Source: CAD feature listing. Evaluate the final solid. Frame: model axes, mm. A direction names the side the tool comes from. Round coordinates to 2 decimals unless told otherwise and drop trailing zeros. Loops run counter-clockwise (first coordinate to the right, second up) from the corner with the lowest first, then second, coordinate; pieces in that order, holes last. Notation, with made-up numbers: (62, 58.25) -> (98, 58.25) arc R6 cw to (98, 66.25) -> close; hole circle Ø3 at (40, 79.25). An arc over 180 degrees is marked (long way). Write item = value, one per line.
from build123d import *

# Parameters (mm, degrees)
SKETCH009_W             = 100.6
SKETCH009_H             = 82.6
PAD006_DEPTH            = 1.6
SKETCH010_W             = 100.6
SKETCH010_H             = 82.6
SKETCH010_W_2           = 98.6
SKETCH010_H_2           = 80.6
PAD007_DEPTH            = 20.6
SKETCH011_W             = 11.5
SKETCH011_H             = 9
PAD008_DEPTH            = 16.6
SKETCH012_W             = 11.5
SKETCH012_H             = 2
PAD009_DEPTH            = 24.3
SKETCH014_R             = 1.75
POCKET004_DEPTH         = 1.6
SKETCH020_W             = 11.5
SKETCH020_H             = 20
PAD013_DEPTH            = 23.9
BODY003_PLACEMENT_ANGLE = 180


with BuildPart() as part:
    # Sketch009 → Pad006 (new body)
    with BuildSketch(Plane.XY):
        Rectangle(SKETCH009_W, SKETCH009_H)
    extrude(amount=PAD006_DEPTH)

    # Sketch010 → Pad007 (join)
    with BuildSketch(Plane.XY):
        Rectangle(SKETCH010_W, SKETCH010_H)
        Rectangle(SKETCH010_W_2, SKETCH010_H_2, mode=Mode.SUBTRACT)
    extrude(amount=PAD007_DEPTH)

    # Sketch011 → Pad008 (join)
    with BuildSketch(Plane.XY):
        with Locations((-41.95, -27.2)):
            Rectangle(SKETCH011_W, SKETCH011_H)
    extrude(amount=PAD008_DEPTH)

    # Sketch012 → Pad009 (join)
    with BuildSketch(Plane.XY):
        with Locations((-41.95, -21.7)):
            Rectangle(SKETCH012_W, SKETCH012_H)
    extrude(amount=PAD009_DEPTH)

    # Sketch014 → Pocket004 (cut)
    with BuildSketch(Plane.XY):
        with Locations((-45, 36)):
            Circle(SKETCH014_R)
        with Locations((11, 36)):
            Circle(SKETCH014_R)
        with Locations((45, 36)):
            Circle(SKETCH014_R)
        with Locations((45, -36)):
            Circle(SKETCH014_R)
        with Locations((11, -36)):
            Circle(SKETCH014_R)
        with Locations((-45, -36)):
            Circle(SKETCH014_R)
    extrude(amount=POCKET004_DEPTH, mode=Mode.SUBTRACT)

    # Sketch020 → Pad013 (join)
    with BuildSketch(Plane.XY):
        with Locations((-41.95, 21.7)):
            Rectangle(SKETCH020_W, SKETCH020_H)
    extrude(amount=PAD013_DEPTH)


with BuildPart() as part_1:
    # Body003 placement: moved
    add(part.part.moved(Location((0, 0, 57.9))).rotate(Axis((0, 0, 57.9), (1, 0, 0)), BODY003_PLACEMENT_ANGLE))


solid = part_1.part
1. Section query A-A (z = 39). Return the cut outline in (x, y).
Evaluation:
outline = (-50.3, -41.3) -> (50.3, -41.3) -> (50.3, 41.3) -> (-50.3, 41.3) -> close; (-47.7, -31.7) -> (-36.2, -31.7) -> (-36.2, -11.7) -> (-47.7, -11.7) -> close; (-47.7, 20.7) -> (-36.2, 20.7) -> (-36.2, 22.7) -> (-47.7, 22.7) -> close; hole (-49.3, -40.3) -> (49.3, -40.3) -> (49.3, 40.3) -> (-49.3, 40.3) -> close
2. Line query: probe 1 along X at (y, z) = (-20, 39); probe 2 along X at (y, z) = (-36, 57.25); probe 3 along Y at (x, z) = (45, 57.3). Output: solid intervals per line, ascending. Write a range as from..to.
Evaluation:
probe_1 = -50.3..-49.3, -47.7..-36.2, 49.3..50.3
probe_2 = -50.3..-46.75, -43.25..9.25, 12.75..43.25, 46.75..50.3
probe_3 = -41.3..-37.75, -34.25..34.25, 37.75..41.3
3. Set-up query: faces 1 (the face through (-43.383, -35.33, 57.111)), 2 (the face through (-49.3, 1, 47)). Return all of +Z, -Z, +X, -X, +Y, -Y with unobstructed straight access to the full face (end or side cutting, diameter ignored); none if empty.
Evaluation:
face_1 = +Z, -Z
face_2 = -Z
4. Mould query, pull axis X, two halves, no side actions, for faces 3 (the face through (-1, -1, 56.3)), 4 (the face through (50.3, 1, 48)), 5 (the face through (-1, 41.3, 48)). Classes: released by +X, released by -X, zero draft, split by the parting line, or undercut.
Evaluation:
face_3 = undercut
face_4 = released by +X
face_5 = zero draft
5. Section query C-C (y = -36). Return the cut outline in (x, z).
Evaluation:
outline = (-50.3, 37.3) -> (-49.3, 37.3) -> (-49.3, 56.3) -> (-46.75, 56.3) -> (-46.75, 57.9) -> (-50.3, 57.9) -> close; (-43.25, 56.3) -> (9.25, 56.3) -> (9.25, 57.9) -> (-43.25, 57.9) -> close; (12.75, 56.3) -> (43.25, 56.3) -> (43.25, 57.9) -> (12.75, 57.9) -> close; (46.75, 56.3) -> (49.3, 56.3) -> (49.3, 37.3) -> (50.3, 37.3) -> (50.3, 57.9) -> (46.75, 57.9) -> close
6. Contact query for flat-ended pins moving along their axis: pin 1 Ø1.5 at (x, z) = (22.5, 36) entering from -Y; pin 2 Ø3.5 at (x, y) = (-42.5, -17.5) entering from -Z; pin 3 Ø2.5 at (x, z) = (-42.5, 36.5) entering from +Y; pin 4 Ø4 at (x, y) = (45, 36) entering from -Z. Output: stop coordinate, or through.
Evaluation:
pin_1 = through
pin_2 = 34
pin_3 = 41.3
pin_4 = 56.3
7. Section query D-D (x = -45). Return the cut outline in (y, z).
Evaluation:
outline = (-41.3, 37.3) -> (-40.3, 37.3) -> (-40.3, 56.3) -> (-37.75, 56.3) -> (-37.75, 57.9) -> (-41.3, 57.9) -> close; (-34.25, 56.3) -> (-31.7, 56.3) -> (-31.7, 34) -> (-11.7, 34) -> (-11.7, 56.3) -> (20.7, 56.3) -> (20.7, 33.6) -> (22.7, 33.6) -> (22.7, 41.3) -> (31.7, 41.3) -> (31.7, 56.3) -> (34.25, 56.3) -> (34.25, 57.9) -> (-34.25, 57.9) -> close; (37.75, 56.3) -> (40.3, 56.3) -> (40.3, 37.3) -> (41.3, 37.3) -> (41.3, 57.9) -> (37.75, 57.9) -> close
8. Section query B-B (x = 45). Return the cut outline in (y, z).
Evaluation:
outline = (-41.3, 37.3) -> (-40.3, 37.3) -> (-40.3, 56.3) -> (-37.75, 56.3) -> (-37.75, 57.9) -> (-41.3, 57.9) -> close; (-34.25, 56.3) -> (34.25, 56.3) -> (34.25, 57.9) -> (-34.25, 57.9) -> close; (37.75, 56.3) -> (40.3, 56.3) -> (40.3, 37.3) -> (41.3, 37.3) -> (41.3, 57.9) -> (37.75, 57.9) -> close
